```python
from build123d import *

# Parameters (mm, degrees)
SKETCH1_W           = 25.4
SKETCH1_H           = 25.4
BOSS_EXTRUDE1_DEPTH = 1.5875
SKETCH2_R           = 0.4953
CUT_EXTRUDE1_DEPTH  = 2.54
SKETCH4_R           = 0.4953
CUT_EXTRUDE2_DEPTH  = 2.54
SKETCH5_W           = 25.4
SKETCH5_H           = 25.4
SKETCH5_R           = 0.4953
CUT_EXTRUDE4_DEPTH  = 0.1016
SKETCH6_R           = 1.27
CUT_EXTRUDE5_DEPTH  = 2.54


with BuildPart() as part:
    # Sketch1 → Boss-Extrude1 (new body)
    with BuildSketch(Plane.XY):
        Rectangle(SKETCH1_W, SKETCH1_H)
    extrude(amount=BOSS_EXTRUDE1_DEPTH)

    # Sketch2 → Cut-Extrude1 (cut)
    with BuildSketch(Plane.XY.offset(1.5875)):
        with Locations((-9.503137046, 5.16324298)):
            Circle(SKETCH2_R)
        with Locations((-6.963137046, 5.16324298)):
            Circle(SKETCH2_R)
        with Locations((-9.503137046, 2.62324298)):
            Circle(SKETCH2_R)
        with Locations((-6.963137046, 2.62324298)):
            Circle(SKETCH2_R)
        with Locations((-9.503137046, 0.08324298)):
            Circle(SKETCH2_R)
        with Locations((-6.963137046, 0.08324298)):
            Circle(SKETCH2_R)
        with Locations((-9.503137046, -2.45675702)):
            Circle(SKETCH2_R)
        with Locations((-6.963137046, -2.45675702)):
            Circle(SKETCH2_R)
        with Locations((-9.503137046, -4.99675702)):
            Circle(SKETCH2_R)
        with Locations((-6.963137046, -4.99675702)):
            Circle(SKETCH2_R)
    extrude(amount=-CUT_EXTRUDE1_DEPTH, mode=Mode.SUBTRACT)

    # Sketch4 → Cut-Extrude2 (cut)
    with BuildSketch(Plane.XY.offset(1.5875)):
        with Locations((7.62, 3.81)):
            Circle(SKETCH4_R)
        with Locations((7.62, 1.27)):
            Circle(SKETCH4_R)
        with Locations((7.62, -1.27)):
            Circle(SKETCH4_R)
        with Locations((9.906, -1.27)):
            Circle(SKETCH4_R)
        with Locations((9.906, 3.81)):
            Circle(SKETCH4_R)
    extrude(amount=-CUT_EXTRUDE2_DEPTH, mode=Mode.SUBTRACT)

    # Sketch5 → Cut-Extrude4 (cut)
    with BuildSketch(Plane.XY.offset(1.5875)):
        Rectangle(SKETCH5_W, SKETCH5_H)
        with BuildLine():
            Line((-5.260680936, 10.015749034), (-8.721290559, 5.586370704))
            ThreePointArc((-8.721290559, 5.586370704), (-10.050460097, 4.46270142), (-9.281723807, 6.024229146))
            Line((-9.281723807, 6.024229146), (-5.607556352, 10.726949034))
            Line((-5.607556352, 10.726949034), (7.041908164, 10.726949034))
            Line((7.041908164, 10.726949034), (11.959875981, 6.884611467))
            Line((11.959875981, 6.884611467), (11.959875981, 2.935863527))
            Line((11.959875981, 2.935863527), (10.380535583, 0.9144))
            Line((10.380535583, 0.9144), (8.434781959, 0.9144))
            ThreePointArc((8.434781959, 0.9144), (6.731, 1.27), (8.434781959, 1.6256))
            Line((8.434781959, 1.6256), (10.033660166, 1.6256))
            Line((10.033660166, 1.6256), (11.248675981, 3.180749326))
            Line((11.248675981, 3.180749326), (11.248675981, 6.53773605))
            Line((11.248675981, 6.53773605), (6.797022365, 10.015749034))
            Line((6.797022365, 10.015749034), (-5.260680936, 10.015749034))
        make_face(mode=Mode.SUBTRACT)
        with BuildLine():
            Line((-8.64215088, 2.401829741), (-7.627203971, 1.60886631))
            Line((-7.627203971, 1.60886631), (1.787159337, 1.60886631))
            Line((1.787159337, 1.60886631), (5.016792936, -0.9144))
            Line((5.016792936, -0.9144), (6.805218041, -0.9144))
            ThreePointArc((6.805218041, -0.9144), (7.62, -0.381), (8.434781959, -0.9144))
            Line((8.434781959, -0.9144), (9.091218041, -0.9144))
            ThreePointArc((9.091218041, -0.9144), (10.795, -1.27), (9.091218041, -1.6256))
            Line((9.091218041, -1.6256), (8.434781959, -1.6256))
            ThreePointArc((8.434781959, -1.6256), (7.62, -2.159), (6.805218041, -1.6256))
            Line((6.805218041, -1.6256), (4.771907137, -1.6256))
            Line((4.771907137, -1.6256), (1.542273539, 0.89766631))
            Line((1.542273539, 0.89766631), (-7.87208977, 0.89766631))
            Line((-7.87208977, 0.89766631), (-9.080009321, 1.841396493))
            ThreePointArc((-9.080009321, 1.841396493), (-10.203678606, 3.170566031), (-8.64215088, 2.401829741))
        make_face(mode=Mode.SUBTRACT)
        with BuildLine():
            Line((9.441579604, 4.622540959), (9.441579604, 6.272789394))
            Line((9.441579604, 6.272789394), (8.487506715, 7.018192829))
            Line((8.487506715, 7.018192829), (7.944356637, 7.018192829))
            Line((7.944356637, 7.018192829), (7.944356637, 6.773792829))
            Line((7.944356637, 6.773792829), (6.794350037, 6.773792829))
            Line((6.794350037, 6.773792829), (6.794350037, 7.973792829))
            Line((6.794350037, 7.973792829), (7.944356637, 7.973792829))
            Line((7.944356637, 7.973792829), (7.944356637, 7.729392829))
            Line((7.944356637, 7.729392829), (8.732392514, 7.729392829))
            Line((8.732392514, 7.729392829), (10.152779604, 6.619664811))
            Line((10.152779604, 6.619664811), (10.152779604, 4.718555699))
            ThreePointArc((10.152779604, 4.718555699), (10.024939422, 2.983486714), (9.441579604, 4.622540959))
        make_face(mode=Mode.SUBTRACT)
        with Locations((-6.963137046, 2.62324298)):
            Circle(SKETCH5_R, mode=Mode.SUBTRACT)
        with BuildLine():
            ThreePointArc((7.196872275, 4.591846487), (8.460566014, 3.520569911), (6.805218041, 3.4544))
            Line((6.805218041, 3.4544), (-5.353507917, 3.4544))
            Line((-5.353507917, 3.4544), (-6.540009321, 4.381396493))
            ThreePointArc((-6.540009321, 4.381396493), (-7.663678606, 5.710566031), (-6.10215088, 4.941829741))
            Line((-6.10215088, 4.941829741), (-5.108622118, 4.1656))
            Line((-5.108622118, 4.1656), (6.587262612, 4.1656))
            Line((6.587262612, 4.1656), (5.292598329, 5.177102595))
            Line((5.292598329, 5.177102595), (-3.586091983, 5.177102595))
            ThreePointArc((-3.586091983, 5.177102595), (-3.889470471, 5.243416559), (-4.025066715, 5.522790336))
            Line((-4.025066715, 5.522790336), (-4.025066715, 7.294419839))
            ThreePointArc((-4.025066715, 7.294419839), (-4.005693121, 7.410191875), (-3.949683339, 7.51334906))
            Line((-3.949683339, 7.51334906), (-3.780891448, 7.729392829))
            Line((-3.780891448, 7.729392829), (-1.732131499, 7.729392829))
            Line((-1.732131499, 7.729392829), (-1.732131499, 7.973792829))
            Line((-1.732131499, 7.973792829), (-0.592131499, 7.973792829))
            Line((-0.592131499, 7.973792829), (-0.592131499, 6.773792829))
            Line((-0.592131499, 6.773792829), (-1.732131499, 6.773792829))
            Line((-1.732131499, 6.773792829), (-1.732131499, 7.018192829))
            Line((-1.732131499, 7.018192829), (-3.313866715, 7.018192829))
            Line((-3.313866715, 7.018192829), (-3.313866715, 5.888302595))
            Line((-3.313866715, 5.888302595), (5.537484128, 5.888302595))
            Line((5.537484128, 5.888302595), (7.196872275, 4.591846487))
        make_face(mode=Mode.SUBTRACT)
        Polygon((4.894350037, 7.729392829), (4.894350037, 7.973792829), (6.034350037, 7.973792829), (6.034350037, 6.773792829), (4.894350037, 6.773792829), (4.894350037, 7.018192829), (1.317875101, 7.018192829), (1.317875101, 6.773792829), (0.167868501, 6.773792829), (0.167868501, 7.973792829), (1.317875101, 7.973792829), (1.317875101, 7.729392829), align=None, mode=Mode.SUBTRACT)
        with Locations((-6.963137046, -2.45675702)):
            Circle(SKETCH5_R, mode=Mode.SUBTRACT)
        with Locations((-9.503137046, 0.08324298)):
            Circle(SKETCH5_R, mode=Mode.SUBTRACT)
        with Locations((-6.963137046, 0.08324298)):
            Circle(SKETCH5_R, mode=Mode.SUBTRACT)
        with Locations((-9.503137046, -4.99675702)):
            Circle(SKETCH5_R, mode=Mode.SUBTRACT)
        with Locations((-6.963137046, -4.99675702)):
            Circle(SKETCH5_R, mode=Mode.SUBTRACT)
        with Locations((-9.503137046, -2.45675702)):
            Circle(SKETCH5_R, mode=Mode.SUBTRACT)
    extrude(amount=-CUT_EXTRUDE4_DEPTH, mode=Mode.SUBTRACT)

    # Sketch6 → Cut-Extrude5 (cut)
    with BuildSketch(Plane(origin=(0, 0, 0), x_dir=(-1, 0, 0), z_dir=(0, 0, -1))):
        with Locations((0, -9.398)):
            Circle(SKETCH6_R)
    extrude(amount=-CUT_EXTRUDE5_DEPTH, mode=Mode.SUBTRACT)


solid = part.part
```
Verification items for the finished model (mm, model axes). Give positions to 0.01 mm unless a question says otherwise; leave off trailing zeros. Loops run counter-clockwise (first coordinate to the right, second up) from the corner with the lowest first, then second, coordinate; pieces in that order, holes last. Notation, with made-up numbers: M 44,43.5 L 82,43.5 A19 ccw 82,78.5 Z; hole C 49.5,5 d11. An arc over 180 degrees is marked long. Return JSON: item names as keys, results as strings.
1) Gauge pin test, flat ends, axial feed: P1, Ø10, axis at x = 7.5, y = 5, coming from the -Z side; P2, Ø6, axis at x = -5, y = -6.5, coming from the +Z side. Record the tip position at first contact, or that the pin passes through.
Findings:
{"P1": "stops at z = 0", "P2": "stops at z = 1.49"}
2) Mould release check, pull along X, two halves, no side actions. Record for faces 1 (the cylindrical face through (-6.49, 5.31, 0.8)), 2 (the flat face through (10, 6, 1.588)), 3 (the flat face through (-12.7, 0, 1)): released by +X, released by -X, zero draft, split by the parting line, or undercut.
Findings:
{"face 1": "undercut", "face 2": "zero draft", "face 3": "released by -X"}
3) Section check B-B, the plane y = -1.27. Count the separate pieces of the cut face and the enclosed holes in it, and give its area (3 significant figures).
Findings:
{"separate pieces": "3", "enclosed holes": "0", "area": "35.3 mm2"}
4) Section check A-A, the plane y = 1.27. Enter the section's corners in (x, z), and give its area (3 significant figures).
Findings:
{"outline": "M -12.7,0 L 7.12,0 L 7.12,1.59 L 6.73,1.59 L 6.73,1.49 L 2.22,1.49 L 2.22,1.59 L -8.35,1.59 L -8.35,1.49 L -12.7,1.49 Z; M 8.12,0 L 12.7,0 L 12.7,1.49 L 10.66,1.49 L 10.66,1.59 L 8.12,1.59 Z", "area": "37.6 mm2"}
5) Material ranges on L1, parallel to Y at x = 0, z = 0.4; L2, parallel to X at y = -2.75, z = 1.1; L3, parallel to Z at x = 11, y = -5.5, recorded low to high. Write a range as [from, to].
Findings:
{"L1": "y = [-12.7, -10.67], [-8.13, 12.7]", "L2": "x = [-12.7, -9.9], [-9.1, -7.36], [-6.56, 12.7]", "L3": "z = [0, 1.49]"}
